from build123d import *

# Parameters (mm, degrees)
CUT_EXTRUDE1_DEPTH = 35
CIRPATTERN1_COUNT  = 30
SKETCH4_W          = 1.5
SKETCH4_H          = 1.584495562


with BuildPart() as part:
    # Sketch1 → Revolve1 (revolve)
    with BuildSketch(Plane(origin=(0, 0, 0), x_dir=(0, 0, -1), z_dir=(1, 0, 0)), mode=Mode.PRIVATE) as revolve1_sk:
        Polygon((0, 6), (40, 6), (40, 21.5), (30, 21.5), (30, 27.25), (0, 27.25), align=None)
    revolve(revolve1_sk.sketch.rotate(Axis((0, 0, 0), (0, 0, -1)), 90), axis=Axis((0, 0, 0), (0, 0, -1)))

    # Sketch2 → Cut-Extrude1 (cut)
    with BuildSketch(Plane.XY):
        with BuildLine():
            Line((3.75, 26.5), (3.674234614, 26.5))
            ThreePointArc((3.674234614, 26.5), (3.199892965, 26.330947502), (2.939387691, 25.9))
            ThreePointArc((2.939387691, 25.9), (2.331759211, 24.612435701), (1.198957881, 23.75))
            Line((1.198957881, 23.75), (-1.198957881, 23.75))
            ThreePointArc((-1.198957881, 23.75), (-2.331759211, 24.612435701), (-2.939387691, 25.9))
            ThreePointArc((-2.939387691, 25.9), (-3.199892965, 26.330947502), (-3.674234614, 26.5))
            Line((-3.674234614, 26.5), (-3.75, 26.5))
            Line((-3.75, 26.5), (-3.75, 28.5))
            Line((-3.75, 28.5), (3.75, 28.5))
            Line((3.75, 28.5), (3.75, 26.5))
        make_face()
    cut_extrude1 = extrude(amount=-CUT_EXTRUDE1_DEPTH, mode=Mode.SUBTRACT)

    # CirPattern1: Cut-Extrude1 ×30 about axis
    cirpattern1_axis = Axis((0, 0, 0), (0, 0, 1))
    for i in range(1, CIRPATTERN1_COUNT):
        add(cut_extrude1.rotate(cirpattern1_axis, i * 360 / CIRPATTERN1_COUNT), mode=Mode.SUBTRACT)

    # Sketch4 → Revolve3 (revolve)
    with BuildSketch(Plane(origin=(0, 0, 0), x_dir=(0, 0, -1), z_dir=(1, 0, 0)), mode=Mode.PRIVATE) as revolve3_sk:
        Polygon((28.5, 25.76477844), (28.5, 25.06477844), (30, 25.06477844), (30, 25.567299693), (29.948888739, 25.376549872), align=None)
        Polygon((30, 25.76477844), (28.5, 25.76477844), (29.948888739, 25.376549872), (30, 25.567299693), align=None)
        Polygon((29.143078062, 28.16477844), (28.5, 25.76477844), (30, 25.76477844), (30, 25.567299693), (30.591966801, 27.776549872), align=None)
        with Locations((29.25, 24.272530659)):
            Rectangle(SKETCH4_W, SKETCH4_H)
        Polygon((0, 25.567299693), (0, 25.76477844), (1.5, 25.76477844), (0.856921938, 28.16477844), (-0.591966801, 27.776549872), align=None)
        Polygon((1.5, 25.06477844), (1.5, 25.76477844), (0.051111261, 25.376549872), (0, 25.567299693), (0, 25.06477844), align=None)
        Polygon((1.5, 25.76477844), (0, 25.76477844), (0, 25.567299693), (0.051111261, 25.376549872), align=None)
        with Locations((0.75, 24.272530659)):
            Rectangle(SKETCH4_W, SKETCH4_H)
    revolve(revolve3_sk.sketch.rotate(Axis((0, 0, 0), (0, 0, 1)), 90), axis=Axis((0, 0, 0), (0, 0, 1)))


solid = part.part
Geometry check sheet. Reference: the model listing, model coordinates, mm. A direction names the side the tool comes from. Round coordinates to 2 decimals unless told otherwise and drop trailing zeros. Loops run counter-clockwise (first coordinate to the right, second up) from the corner with the lowest first, then second, coordinate; pieces in that order, holes last.
Item 1: Cross-section at A-A on x = 0. Record the boundary of the cut face in (y, z).
Item 2: Gauge pin test, flat ends, axial feed: pin 1 (1.5 mm diameter, centred on x = -3.5, z = -26, fed in from -Y); pin 2 (1 mm diameter, centred on x = -21.5, y = -2, fed in from +Z); pin 3 (5 mm diameter, centred on y = -22, z = -9, fed in from -X); pin 4 (3 mm diameter, centred on x = -18.5, y = 19, fed in from +Z). Record the tip position at first contact, or that the pin passes through.
Item 3: Access from +Z, -Z, +X, -X, +Y, -Y to the whole of each face (thin tool, end or side, straight path). Record for faces 1 (the flat face through (20.56, -11.89, -14.81)), 2 (the cylindrical face through (-7.04, -23.34, -14.81)), 3 (the cylindrical face through (-3.06, 24.19, -14.81)), 4 (the cylindrical face through (-8.022, 23.025, -14.811)).
Item 4: Thickness scan on line 1 (Y direction, x = 0, z = -11); line 2 (Z direction, x = -22.5, y = 8); line 3 (Z direction, x = 1.5, y = 11). Record the ranges inside material, lowest first.
Answer sheet:
1. outline: (-28.16, -29.14) - (-27.78, -30.59) - (-25.57, -30) - (-21.5, -30) - (-21.5, -40) - (-6, -40) - (-6, 0) - (-25.57, 0) - (-27.78, 0.59) - (-28.16, -0.86) - (-25.76, -1.5) - (-23.75, -1.5) - (-23.75, -28.5) - (-25.76, -28.5) - close; (6, -40) - (21.5, -40) - (21.5, -30) - (25.57, -30) - (27.78, -30.59) - (28.16, -29.14) - (25.76, -28.5) - (23.75, -28.5) - (23.75, -1.5) - (25.76, -1.5) - (28.16, -0.86) - (27.78, 0.59) - (25.57, 0) - (6, 0) - close
2. pin 1: stops at y = -24.74
2. pin 2: stops at z = 0
2. pin 3: stops at x = -13.57
2. pin 4: stops at z = 0.59
3. face 1: +X
3. face 2: -Y
3. face 3: +Y
3. face 4: -X, +Y
4. line 1: y = -23.75 to -6, 6 to 23.75
4. line 2: z = -30 to -28.5, -1.5 to 0
4. line 3: z = -40 to 0
